Work out the finished part from the listing and answer in its coordinate system (mm). Face numbers are marked on the shaded views. A direction names the side the tool comes from. Give positions to 0.01 mm unless a question says otherwise; leave off trailing zeros. Loops run counter-clockwise (first coordinate to the right, second up) from the corner with the lowest first, then second, coordinate; pieces in that order, holes last. Notation, with made-up numbers: M -18,-15.75 L 34,-15.75 A22 ccw 34,-6.75 Z; hole C 51.5,1 d1. An arc over 180 degrees is marked long. Use a Markdown table: item, result.
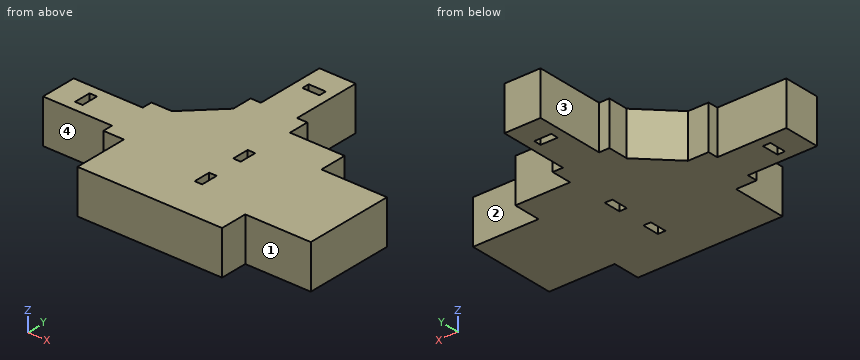
Autodesk Inventor part; units mm, degrees
ref_plane "YZ Plane" through (0, 0, 0) normal (1, 0, 0) x (0, 1, 0)
ref_plane "XZ Plane" through (0, 0, 0) normal (0, 1, 0) x (-1, 0, 0)
ref_plane "XY Plane" through (0, 0, 0) normal (0, 0, 1) x (1, 0, 0)
sketch "Sketch1" plane through (0, 0, 0) normal (0, 0, 1) x (1, 0, 0)
  line L0 (-2.6473, 22.1) -> (2.6473, 22.1)
  line L1 (2.6473, 22.1) -> (2.6473, 12)
  line L2 (2.6473, 12) -> (4.1473, 12)
  line L3 (4.1473, 12) -> (4.1473, 9)
  line L4 (4.1473, 9) -> (12.1473, 9)
  line L5 (0, 22.1) -> (0, 0) construction
  line L6 (-2.6473, 22.1) -> (-2.6473, 12)
  line L7 (-2.6473, 12) -> (-4.1473, 12)
  line L8 (-1.25, 18.6) -> (1.25, 18.6)
  line L9 (1.25, 18.6) -> (1.25, 17.5)
  line L10 (1.25, 17.5) -> (-1.25, 17.5)
  line L11 (-1.25, 17.5) -> (-1.25, 18.6)
  line L12 (-5, -12.1473) -> (12.1473, -12.1473)
  line L13 (12.1473, 9) -> (12.1473, 5)
  line L14 (12.1473, 5) -> (21.7323, 5)
  line L15 (21.7323, -8.1473) -> (12.1473, -8.1473)
  line L16 (12.1473, -8.1473) -> (12.1473, -12.1473)
  line L17 (3.0473, 3) -> (4.1473, 3)
  line L18 (4.1473, 3) -> (4.1473, 0.5)
  line L19 (4.1473, 0.5) -> (3.0473, 0.5)
  line L20 (3.0473, 0.5) -> (3.0473, 3)
  line L21 (-4.1473, 12) -> (-19.8527, 12) construction
  line L22 (0, 0) -> (-12, 12) construction
  line L23 (-22.1, 2.6473) -> (-22.1, -2.6473)
  line L24 (-22.1, -2.6473) -> (-12, -2.6473)
  line L25 (-12, -2.6473) -> (-12, -4.1473)
  line L26 (-12, -4.1473) -> (-9, -4.1473)
  line L27 (-9, -4.1473) -> (-9, -12.1473)
  line L28 (-22.1, 2.6473) -> (-12, 2.6473)
  line L29 (-12, 2.6473) -> (-12, 4.1473)
  line L30 (-18.6, 1.25) -> (-18.6, -1.25)
  line L31 (-18.6, -1.25) -> (-17.5, -1.25)
  line L32 (-17.5, -1.25) -> (-17.5, 1.25)
  line L33 (-17.5, 1.25) -> (-18.6, 1.25)
  line L34 (-9, -12.1473) -> (-5, -12.1473)
  line L35 (-12, 12) -> (-12, -12.1473) construction
  line L36 (-4.1473, 12) -> (-4.1473, 9)
  line L37 (-9, 4.1473) -> (-12, 4.1473)
  line L38 (-4.1473, 9) -> (-9, 4.1473)
  line L39 (21.7323, 5) -> (21.7323, -8.1473)
  line L40 (21.7323, -1.5737) -> (3.3412, -1.5737) construction
  line L41 (3.0473, -6.1473) -> (4.1473, -6.1473)
  line L42 (4.1473, -6.1473) -> (4.1473, -3.6473)
  line L43 (4.1473, -3.6473) -> (3.0473, -3.6473)
  line L44 (3.0473, -3.6473) -> (3.0473, -6.1473)
  line L45 (-22.1, 0) -> (21.7323, 0) construction
  point P0 (0, 17.5)
  point P1 (3.0473, 1.75)
  point P2 (-17.5, 0)
  point P3 (4.1473, 1.75)
  point P4 (4.1473, 10.5)
  dimension "d4" = 1.5
  dimension "d5" = 3
  dimension "d26" = 10.1
  dimension "d27" = 5.2946
  dimension "d31" = 2.5
  dimension "d32" = 1.1
  dimension "d35" = 5.5
  dimension "d37" = 9.585
  dimension "d41" = 1.1
  dimension "d42" = 2.5
  dimension "d45" = 2
  dimension "d61" = 45
  dimension "d70" = 8
  dimension "d72" = 12
  dimension "BearingShaftOffset" = 1.5737
  dimension "BearingHolderHeight" = 23.6737
  dimension "LatchHeight" = 13.1473
  dimension "d95" = 24.1473
extrude "Extrusion2" add sketch "Sketch1" along normal blind 6.39
equation "\"BearingDiameter\" = 24"
equation "\"WoodThickness\" = 6.39"
equation "\"BearingWidth\" = 7"
equation "\"BearingShaftDiameter\" = 8"
equation "\"ZipTieWidth\" = 2.5"
equation "\"ZipTieThickness\" = 1.1"
equation "\"ZipTieClearance\" = 1"
equation "\"ZipTieDistance\" = 10"
equation "\"BearingSiliconeWidth\" = 13.2"
properties part number "BearingStand" material "MDF Medium Density Fiberboard"
(1) Consider probe 1 along Y at (x, z) = (4, 2.5); probe 2 along X at (y, z) = (1, 1.5); probe 3 along X at (y, z) = (-5.5, 4.75). Determine where each line is inside the solid, lowest interval first. Write a range as [from, to].
Entries:
| item | result |
|---|---|
| probe 1 | y = [-12.15, -6.15], [-3.65, 0.5], [3, 12] |
| probe 2 | x = [-22.1, -18.6], [-17.5, 3.05], [4.15, 21.73] |
| probe 3 | x = [-9, 3.05], [4.15, 21.73] |
(2) Which of the six approach directions +Z, -Z, +X, -X, +Y, -Y give full straight-line access (tool end or side, diameter ignored) to the marked faces 1, 2, 3 and 4?
Entries:
| item | result |
|---|---|
| face 1 | +Z, -Z, +X, -Y |
| face 2 | +Z, -Z, +X, +Y |
| face 3 | +Z, -Z, -X, +Y |
| face 4 | +Z, -Z, -X, -Y |
(3) A cutting plane is placed at A-A (z = 3). Count the separate pieces of the cut face and the enclosed holes in it, and give its area (3 significant figures).
Entries:
| item | result |
|---|---|
| separate pieces | 1 |
| enclosed holes | 4 |
| area | 707 mm² |
(4) Given P1, Ø3.5, axis at x = -10.5, z = 3, coming from the +Y side; P2, Ø1.2, axis at x = 3.5, z = 2.5, coming from the +Y side; P3, Ø1.9, axis at x = -17, z = 5, coming from the -Y side, each flat-ended and moving along its own axis, determine where each tip first touches the part or whether it passes through.
Entries:
| item | result |
|---|---|
| P1 | stops at y = 4.4 |
| P2 | stops at y = 12 |
| P3 | stops at y = -2.65 |
(5) A cutting plane is placed at B-B (y = 9.5). Write down the section's boundary in (x, z), and give its area (3 significant figures).
Entries:
| item | result |
|---|---|
| outline | M -4.15,0 L 4.15,0 L 4.15,6.39 L -4.15,6.39 Z |
| area | 53.0 mm² |
